Geometry: final body of the model. Coordinates: model frame, mm. Face numbers are marked on the shaded views. Round coordinates to 2 decimals unless told otherwise and drop trailing zeros. Loops run counter-clockwise (first coordinate to the right, second up) from the corner with the lowest first, then second, coordinate; pieces in that order, holes last. Notation, with made-up numbers: M 4,61 L 16,61 A18 cw 16,72 Z; hole C -28.75,22.25 d5. An arc over 180 degrees is marked long. Write each question's results on one line, items separated by ' | '.
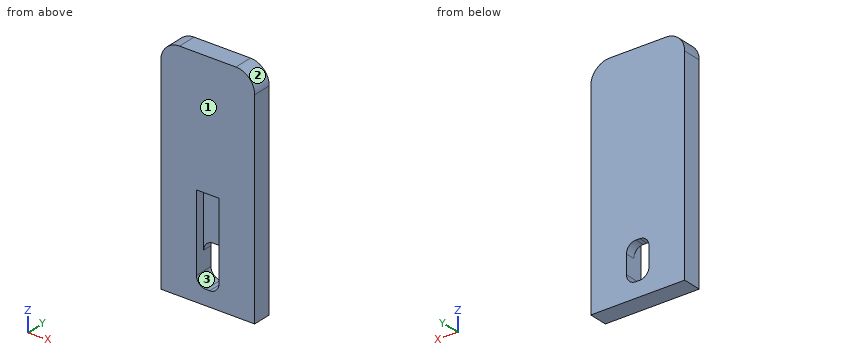
```python
from build123d import *

# Parameters (mm, degrees)
F1_DEPTH = 10
F3_DEPTH = 11
F4_W     = 12
F4_H     = 33.18387
F5_DEPTH = 5


with BuildPart() as f1:
    # F0 (on Front) → F1 (new body)
    with BuildSketch(Plane.XZ):
        with BuildLine():
            ThreePointArc((25, 50), (22.071068, 57.071068), (15, 60))
            Line((15, 60), (-15, 60))
            ThreePointArc((-15, 60), (-22.071068, 57.071068), (-25, 50))
            Line((-25, 50), (-25, -60))
            Line((-25, -60), (25, -60))
            Line((25, -60), (25, 50))
        make_face()
    extrude(amount=F1_DEPTH)

    # F2 (on face) → F3 (cut)
    with BuildSketch(Plane.XZ.offset(10)):
        with BuildLine():
            Line((1, -32.074185), (-1, -32.074185))
            ThreePointArc((-1, -32.074185), (-4.535534, -33.538651), (-6, -37.074185))
            Line((-6, -37.074185), (-6, -47.074185))
            ThreePointArc((-6, -47.074185), (-4.535534, -50.609719), (-1, -52.074185))
            Line((-1, -52.074185), (1, -52.074185))
            ThreePointArc((1, -52.074185), (4.535534, -50.609719), (6, -47.074185))
            Line((6, -47.074185), (6, -37.074185))
            ThreePointArc((6, -37.074185), (4.535534, -33.538651), (1, -32.074185))
        make_face()
    extrude(amount=-F3_DEPTH, mode=Mode.SUBTRACT)

    # F4 (on face) → F5 (cut)
    with BuildSketch(Plane.XZ.offset(10)):
        with Locations((0, -22.583467)):
            Rectangle(F4_W, F4_H)
    extrude(amount=-F5_DEPTH, mode=Mode.SUBTRACT)


solid = f1.part
```
1. Draft query along X for the marked faces 1, 2 and 3. Return one class per face: pulls with the +X half, pulls with the -X half, needs draft (parallel to the pull), parting line crosses it, or undercut.
Answer key:
face 1: needs draft | face 2: pulls with the +X half | face 3: undercut
2. Section C-C (y = -2.25). Output: boundary loops of the cut face in (x, z).
Answer key:
outline: M -25,-60 L 25,-60 L 25,50 A10 ccw 15,60 L -15,60 A10 ccw -25,50 Z; hole M -6,-47.07 A5 ccw -1,-52.07 L 1,-52.07 A5 ccw 6,-47.07 L 6,-37.07 A5 ccw 1,-32.07 L -1,-32.07 A5 ccw -6,-37.07 Z
3. Section A-A (y = -8.75). Output: boundary loops of the cut face in (x, z).
Answer key:
outline: M -25,-60 L 25,-60 L 25,50 A10 ccw 15,60 L -15,60 A10 ccw -25,50 Z; hole M -6,-47.07 A5 ccw -1,-52.07 L 1,-52.07 A5 ccw 6,-47.07 L 6,-5.99 L -6,-5.99 Z
4. Pin query (flat end, axial travel): P1, Ø4, axis at x = -1.5, z = -27.5, coming from the -Y side. Return the tip coordinate at first contact, or that it passes through.
Answer key:
P1: stops at y = -5
5. Section B-B (x = -4). Output: boundary loops of the cut face in (y, z), then the cut area to 3 significant figures.
Answer key:
outline: M -10,-60 L 0,-60 L 0,-51.07 L -10,-51.07 Z; M -10,-5.99 L -5,-5.99 L -5,-33.07 L 0,-33.07 L 0,60 L -10,60 Z | area: 885 mm²
6. Ray query, probe 1 along X at (y, z) = (-8.25, -46.5); probe 2 along Z at (x, y) = (-2, -8.25); probe 3 along Z at (x, y) = (3.5, -4.5). Return the intervals inside material, ascending.
Answer key:
probe 1: x = -25 to -6, 6 to 25 | probe 2: z = -60 to -51.97, -5.99 to 60 | probe 3: z = -60 to -51.4, -32.74 to 60
